Part print with two shaded views. Sizes in mm from the minimum x, y, z corner. A direction names the side the tool comes from. Coordinates: 2 decimals unless noted, no trailing zeros. Loops run counter-clockwise (first coordinate to the right, second up) from the corner with the lowest first, then second, coordinate; pieces in that order, holes last. Notation, with made-up numbers: (51, 76) -> (84, 76) arc R29 ccw to (84, 114) -> close; hole circle Ø6 at (-6.5, 45.5). An arc over 180 degrees is marked (long way). Use one line per item in the form item = value.
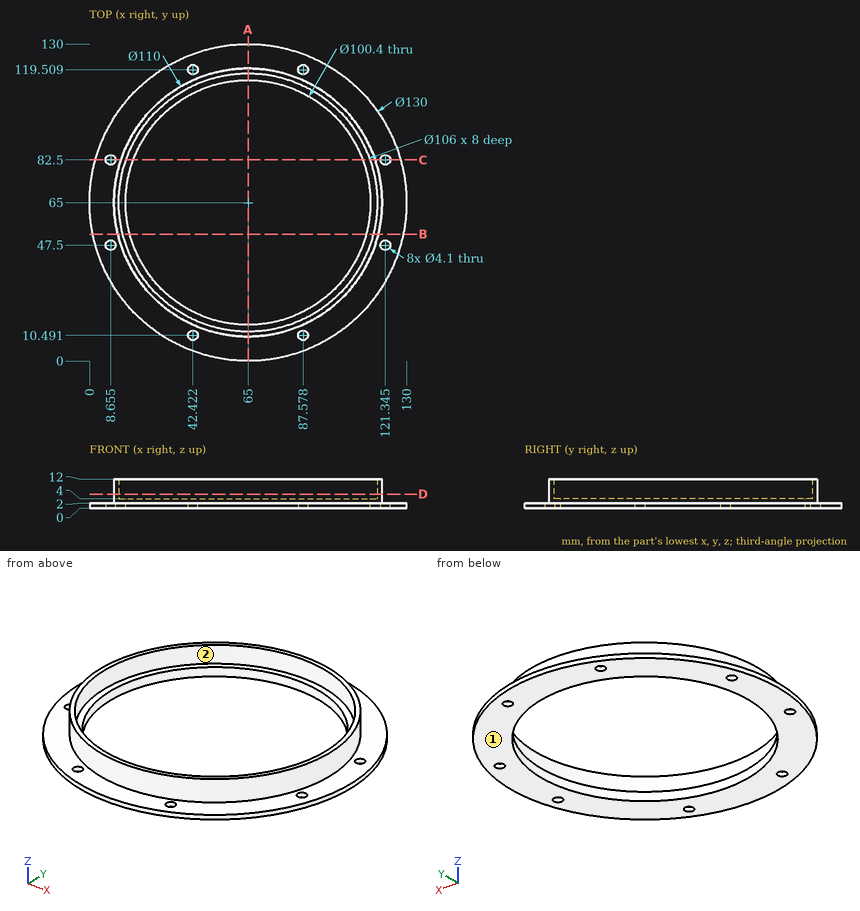
Q1. Wall check: line 1 along X through (y, z) = (66, 4.75); line 2 along X through (y, z) = (36, 1.75) (1 decimal). Give the ranges that are in metal, low to high.
Result:
line_1 = 10.01 to 12.01, 117.99 to 119.99
line_2 = 6.8 to 24, 106 to 123.2
Q2. Which spindle directions (+Z, -Z, +X, -X, +Y, -Y) get a long thin tool onto all of the face, cutting with end or side? Do the marked faces 1 and 2. Say none if no direction does.
Result:
face_1 = -Z, +X, -X, +Y, -Y
face_2 = +Z
Q3. Band-saw the part on C-C, the plane y = 82.5. Write the cut outline in (x, z) (1 decimal).
Result:
outline = (2.4, 0) -> (6.6, 0) -> (6.6, 2) -> (2.4, 2) -> close; (10.7, 0) -> (17.9, 0) -> (17.9, 4) -> (15, 4) -> (15, 12) -> (12.9, 12) -> (12.9, 2) -> (10.7, 2) -> close; (112.1, 0) -> (119.3, 0) -> (119.3, 2) -> (117.1, 2) -> (117.1, 12) -> (115, 12) -> (115, 4) -> (112.1, 4) -> close; (123.4, 0) -> (127.6, 0) -> (127.6, 2) -> (123.4, 2) -> close
Q4. Band-saw the part on A-A, the plane x = 65. Write the cut outline in (y, z).
Result:
outline = (0, 0) -> (14.8, 0) -> (14.8, 4) -> (12, 4) -> (12, 12) -> (10, 12) -> (10, 2) -> (0, 2) -> close; (115.2, 0) -> (130, 0) -> (130, 2) -> (120, 2) -> (120, 12) -> (118, 12) -> (118, 4) -> (115.2, 4) -> close
Q5. Pin check, flat tips, straight feed: pin 1 Ø3 at (x, z) = (19, 10.5) entering from -Y; pin 2 Ø1 at (x, z) = (53, 4) entering from +Y; pin 3 Ø5.5 at (x, y) = (42.42, 10.49) entering from +Z. Stop position of each tip, or through.
Result:
pin_1 = 32.68
pin_2 = 118.78
pin_3 = 2
Q6. Band-saw the part on B-B, the plane y = 52. Write the cut outline in (x, z), and give its area (3 significant figures).
Result:
outline = (1.31, 0) -> (16.51, 0) -> (16.51, 4) -> (13.62, 4) -> (13.62, 12) -> (11.56, 12) -> (11.56, 2) -> (1.31, 2) -> close; (113.49, 0) -> (128.69, 0) -> (128.69, 2) -> (118.44, 2) -> (118.44, 12) -> (116.38, 12) -> (116.38, 4) -> (113.49, 4) -> close
area = 114 mm2
Q7. Band-saw the part on D-D, the plane z = 5.75. Write the cut outline in (x, y).
Result:
outline = circle Ø110 at (65, 65); hole circle Ø106 at (65, 65)
